```python
from build123d import *

# Parameters (mm, degrees)
CROQUIS1_R              = 113.228412481
CROQUIS1_R_2            = 30
CROQUIS1_R_3            = 10
SALIENTE_EXTRUIR2_DEPTH = 20
SALIENTE_EXTRUIR3_DEPTH = 8


with BuildPart() as part:
    # Croquis1 → Saliente-Extruir2 (new body)
    with BuildSketch(Plane(origin=(0, 0, 0), x_dir=(1, 0, 0), z_dir=(0, 1, 0))):
        with Locations(Location((0, 0, 0), (0, 0, 270))):
            Circle(CROQUIS1_R)
        with Locations(Location((0, 79.050232258, 0), (0, 0, 270))):
            Circle(CROQUIS1_R_2, mode=Mode.SUBTRACT)
        with Locations(Location((68.459509311, 39.525116129, 0), (0, 0, 270))):
            Circle(CROQUIS1_R_2, mode=Mode.SUBTRACT)
        with Locations(Location((68.459509311, -39.525116129, 0), (0, 0, 270))):
            Circle(CROQUIS1_R_2, mode=Mode.SUBTRACT)
        with Locations(Location((0, -79.050232258, 0), (0, 0, 270))):
            Circle(CROQUIS1_R_2, mode=Mode.SUBTRACT)
        with Locations(Location((-68.459509311, -39.525116129, 0), (0, 0, 270))):
            Circle(CROQUIS1_R_2, mode=Mode.SUBTRACT)
        with Locations(Location((-68.459509311, 39.525116129, 0), (0, 0, 270))):
            Circle(CROQUIS1_R_2, mode=Mode.SUBTRACT)
        with Locations(Location((0, 0, 0), (0, 0, 270))):
            Circle(CROQUIS1_R_3, mode=Mode.SUBTRACT)
    extrude(amount=SALIENTE_EXTRUIR2_DEPTH)

    # Croquis2 → Saliente-Extruir3 (add)
    with BuildSketch(Plane.XZ):
        Polygon((113.057016297, -6.227716999), (113.651716101, 5.197666723), (104.054393451, 11.425383723), (93.862370997, 6.227716999), (93.267671193, -5.197666723), (102.864993843, -11.425383723), align=None)
    extrude(amount=SALIENTE_EXTRUIR3_DEPTH)


solid = part.part
```
For this review, take the finished solid that the model builds, in its own axes (mm). A direction names the side the tool comes from. Coordinates: 2 decimals unless noted, no trailing zeros. Write each loop counter-clockwise with the first axis right and the second up, starting at its lowest first coordinate (ties: lowest second). Pieces come first, ordered by that corner, then holes.
(1) Add section D-D on z = -29. Give the boundary of the cut face in (x, y), then the cut area to 3 significant figures.
(2) Add section B-B on z = -57.5. Give the boundary of the cut face in (x, y), then the cut area to 3 significant figures.
(3) Wall thickness on probe 1 along Z at (x, y) = (12.5, 14); probe 2 along X at (y, z) = (3.5, 41.5); probe 3 along X at (y, z) = (12.75, 0): over which ranges is each line inside the solid? List them lowest first.
(4) Add section C-C on x = 87. Give the boundary of the cut face in (y, z).
(5) Add section A-A on x = 0. Give the boundary of the cut face in (y, z).
(6) For pin 1 Ø6 at (x, y) = (-62, 3.5) entering from +Z; pin 2 Ø1 at (x, y) = (10, 16) entering from +Z; pin 3 Ø1.5 at (y, z) = (5, -13) entering from +X, all flat-tipped, find the tip position at first contact; note any pin that passes through.
(7) The part is to be moulded in two halves that separate along Z. For faces 1 (the face through (-68.9, 9.86, -89.85)), 2 (the face through (108.92, -3.94, 8.27)), 3 (the face through (-9.76, 9.86, -2.17)), say which applies: +Z half, -Z half, draft (parallel to the pull), parting line (faces both ways), or undercut.
(8) Tool access review of faces 4 (the face through (98, -3.94, -8.27)), 5 (the face through (107.89, -3.944, -8.863)), 6 (the face through (93.57, -3.94, 0.6)): name each direction out of +Z, -Z, +X, -X, +Y, -Y from which nothing blocks a thin tool from reaching the whole face with its end or side.
Answer sheet:
1. outline: (-109.45, 0) - (-96.55, 0) - (-96.55, 20) - (-109.45, 20) - close; (-40.37, 0) - (40.37, 0) - (40.37, 20) - (-40.37, 20) - close; (96.55, 0) - (109.45, 0) - (109.45, 20) - (96.55, 20) - close
1. area: 2,130 mm2
2. outline: (-97.54, 0) - (-92.48, 0) - (-92.48, 20) - (-97.54, 20) - close; (-44.44, 0) - (-20.87, 0) - (-20.87, 20) - (-44.44, 20) - close; (20.87, 0) - (44.44, 0) - (44.44, 20) - (20.87, 20) - close; (92.48, 0) - (97.54, 0) - (97.54, 20) - (92.48, 20) - close
2. area: 1,150 mm2
3. probe 1: z = -112.54 to -106.32, -51.78 to 51.78, 106.32 to 112.54
3. probe 2: x = -105.35 to -98.39, -38.52 to 38.52, 98.39 to 105.35
3. probe 3: x = -113.23 to -10, 10 to 113.23
4. outline: (0, -72.47) - (20, -72.47) - (20, -63.11) - (0, -63.11) - close; (0, -15.94) - (20, -15.94) - (20, 15.94) - (0, 15.94) - close; (0, 63.11) - (20, 63.11) - (20, 72.47) - (0, 72.47) - close
5. outline: (0, -113.23) - (20, -113.23) - (20, -109.05) - (0, -109.05) - close; (0, -49.05) - (20, -49.05) - (20, -10) - (0, -10) - close; (0, 10) - (20, 10) - (20, 49.05) - (0, 49.05) - close; (0, 109.05) - (20, 109.05) - (20, 113.23) - (0, 113.23) - close
6. pin 1: stops at z = 96.64
6. pin 2: stops at z = 112.83
6. pin 3: stops at x = 112.56
7. face 1: parting line
7. face 2: +Z half
7. face 3: undercut
8. face 4: -Z, -X, -Y
8. face 5: -Z, +X, -Y
8. face 6: +Z, -X, -Y
